```python
from build123d import *

# Parameters (mm, degrees)
SKETCH2_W           = 100
SKETCH2_H           = 64
BOSS_EXTRUDE1_DEPTH = 22
CUT_EXTRUDE1_DEPTH  = 126
SKETCH4_W           = 15
SKETCH4_H           = 64
BOSS_EXTRUDE2_DEPTH = 75
CHAMFER1_SIZE       = 16
CHAMFER2_SIZE       = 16
RIB2_REACH          = 128.044
SKETCH10_WALL_W     = 322.09589175
SKETCH10_WALL_H     = 12


with BuildPart() as part:
    # Sketch2 → Boss-Extrude1 (new body)
    with BuildSketch(Plane(origin=(0, 0, 0), x_dir=(1, 0, 0), z_dir=(0, 1, 0))):
        with Locations((-23.852270783, -4.169452289)):
            Rectangle(SKETCH2_W, SKETCH2_H)
    extrude(amount=BOSS_EXTRUDE1_DEPTH)

    # Sketch3 → Cut-Extrude1 (cut)
    with BuildSketch(Plane.ZY.offset(73.852270783)):
        Polygon((19.169452289, 12.073281473), (12.217656655, 0), (-3.860035403, 0), (-10.830547711, 12.073281473), align=None)
    extrude(amount=-CUT_EXTRUDE1_DEPTH, mode=Mode.SUBTRACT)

    # Sketch4 → Boss-Extrude2 (add)
    with BuildSketch(Plane(origin=(0, 22, 0), x_dir=(1, 0, 0), z_dir=(0, 1, 0))):
        with Locations((-66.352270783, -4.169452289)):
            Rectangle(SKETCH4_W, SKETCH4_H)
    extrude(amount=BOSS_EXTRUDE2_DEPTH)

    # Chamfer1
    chamfer1_edges = [part.edges().sort_by_distance(p)[0] for p in [
        (-66.352270783, 97, 36.169452289),
    ]]
    chamfer(chamfer1_edges, length=CHAMFER1_SIZE)

    # Chamfer2
    chamfer2_edges = [part.edges().sort_by_distance(p)[0] for p in [
        (-66.352270783, 97, -27.830547711),
    ]]
    chamfer(chamfer2_edges, length=CHAMFER2_SIZE)

    # Sketch10 wall → Rib2 (add, up to next)
    with BuildSketch(Plane(origin=(-31.352270783, 42, 4.169452289), x_dir=(0.808736084303, -0.588171697675, 0), z_dir=(0.588171697675, 0.808736084303, 0)), mode=Mode.PRIVATE) as rib2_sk1:
        Rectangle(SKETCH10_WALL_W, SKETCH10_WALL_H)
    rib2_tool1 = extrude(rib2_sk1.sketch, amount=-RIB2_REACH, mode=Mode.PRIVATE) - part.part
    add(rib2_tool1.solids().sort_by_distance((-31.352270783, 42, 4.169452289))[0])


solid = part.part
```
Can you work these out from the model? Positions are in its coordinate system, mm. A direction names the side the tool comes from. Give positions to 0.01 mm unless a question says otherwise; leave off trailing zeros. Write each loop counter-clockwise with the first axis right and the second up, starting at its lowest first coordinate (ties: lowest second). Pieces come first, ordered by that corner, then holes. Notation, with made-up numbers: (2, 15) - (10, 15) arc R29 cw to (10, 45) - close; hole circle Ø10 at (79.25, -36). An arc over 180 degrees is marked (long way). Write item = value, one per line. Start each with the question number.
1. For pin 1 (6 mm diameter, centred on y = 79, z = -1.5, fed in from +X); pin 2 (2 mm diameter, centred on y = 43, z = 8, fed in from +X); pin 3 (4 mm diameter, centred on x = -49, z = -14.5, fed in from +Y); pin 4 (9 mm diameter, centred on x = -29, z = -0.5, fed in from -Y), each with a flat end and sliding along its axis, tell me the tip position at first contact or that it passes through.
2. Imagine slicing it at B-B (z = 17). Please give me the cut outline in (x, y).
3. Imagine slicing it at D-D (z = 27). Please give me the cut outline in (x, y).
4. Please list where these lines run through material, in increasing order: line 1 (Y direction, x = -48, z = 27); line 2 (Y direction, x = 5, z = 9); line 3 (Z direction, x = -55, y = 52.5).
5. Imagine slicing it at C-C (y = 47). Please give me the cut outline in (x, z), and give its area (3 significant figures).
6. Thinking about a two-plate mould opening in Z: for faces 5 (the face through (-24.55, 6.12, 15.74)), 6 (the face through (-39, 32, -1.831)), 7 (the face through (-73.852, 48, 5)), 8 (the face through (-24.552, 5.952, -7.296)), which applies, released by +Z, released by -Z, zero draft, split by the parting line, or undercut?
7. Imagine slicing it at A-A (x = 16.5). Please give me the cut outline in (y, z), and give its area (3 significant figures).
8. On a 3-axis mill with a long thin cutter (end or side, diameter ignored), from which of +Z, -Z, +X, -X, +Y, -Y can I reach the whole of each face in a straight line? I mean faces 1 (the face through (-39, 32, 10.169)), 2 (the face through (-17, 22, -3)), 3 (the face through (-25, 12.073, 4)), 4 (the face through (-66.46, 88.89, -19.94)). Say none if no direction works.
Worked answers:
q1.pin_1 = -58.85
q1.pin_2 = -31.35
q1.pin_3 = 22
q1.pin_4 = 0
q2.outline = (-73.85, 0) - (26.15, 0) - (26.15, 8.31) - (-73.85, 8.31) - close; (-73.85, 12.07) - (26.15, 12.07) - (26.15, 22) - (-58.85, 22) - (-58.85, 97) - (-73.85, 97) - close
q3.outline = (-73.85, 0) - (26.15, 0) - (26.15, 22) - (-58.85, 22) - (-58.85, 90.17) - (-73.85, 90.17) - close
q4.line_1 = 0 to 22
q4.line_2 = 12.07 to 22
q4.line_3 = -1.83 to 10.17
q5.outline = (-73.85, -27.83) - (-58.85, -27.83) - (-58.85, -1.83) - (-38.23, -1.83) - (-38.23, 10.17) - (-58.85, 10.17) - (-58.85, 36.17) - (-73.85, 36.17) - close
q5.area = 1,210 mm2
q6.face_5 = undercut
q6.face_6 = released by -Z
q6.face_7 = zero draft
q6.face_8 = undercut
q7.outline = (0, -27.83) - (22, -27.83) - (22, 36.17) - (0, 36.17) - (0, 12.22) - (12.07, 19.17) - (12.07, -10.83) - (0, -3.86) - close
q7.area = 1,130 mm2
q8.face_1 = +Z, +X, +Y
q8.face_2 = +X, +Y
q8.face_3 = +X, -X
q8.face_4 = -Z, +X, -X, +Y
